from build123d import *

# Parameters (mm, degrees)
F0_W          = 70
F0_H          = 50
F1_DEPTH      = 130
F1_DEPTH_BACK = 70
F3_DEPTH      = 3


with BuildPart() as f1:
    # F0 (on Front) → F1 (new body, two sides)
    with BuildSketch(Plane.XZ) as f1_sk:
        Rectangle(F0_W, F0_H)
    extrude(amount=F1_DEPTH)
    extrude(f1_sk.sketch, amount=-F1_DEPTH_BACK)

    # F2 (on face) → F3 (join)
    with BuildSketch(Plane.XY.offset(25)):
        Polygon((-20, -117.372043), (0, -117.372043), (19.486902, -117.372043), (19.486902, -97.372043), (17.486902, -97.372043), (17.486902, -115.372043), (1, -115.372043), (1, -97.372043), (-1, -97.372043), (-1, -115.372043), (-18, -115.372043), (-18, -97.372043), (-20, -97.372043), align=None)
        with BuildLine():
            Line((8.707276, -43.856528), (19.913864, -43.856528))
            Line((19.913864, -43.856528), (19.913864, -41.856528))
            Line((19.913864, -41.856528), (4.924431, -41.856528))
            ThreePointArc((4.924431, -41.856528), (4.807975, -38.322004), (5.569528, -34.868535))
            Line((5.569528, -34.868535), (19.913864, -25.94221))
            Line((19.913864, -25.94221), (19.913864, -23.94221))
            Line((19.913864, -23.94221), (16.171332, -26.208643))
            ThreePointArc((16.171332, -26.208643), (16.198489, -26.228568), (16.225597, -26.24856))
            ThreePointArc((16.225597, -26.24856), (16.190659, -26.233277), (16.155661, -26.218133))
            Line((16.155661, -26.218133), (4.924431, -33.019635))
            ThreePointArc((4.924431, -33.019635), (-12.74275, -26.189347), (-19.573038, -43.856528))
            Line((-19.573038, -43.856528), (8.220368, -43.856528))
            ThreePointArc((8.220368, -43.856528), (8.255555, -43.764356), (8.290131, -43.671953))
            ThreePointArc((8.290131, -43.671953), (8.497604, -43.766725), (8.707276, -43.856528))
        make_face()
        with BuildLine():
            ThreePointArc((-17.680509, -41.856528), (-7.511621, -26.91543), (2.657267, -41.856528))
            Line((2.657267, -41.856528), (-17.680509, -41.856528))
        make_face(mode=Mode.SUBTRACT)
        with BuildLine():
            Line((-17.549662, 0), (-19.378563, 0))
            ThreePointArc((-19.378563, 0), (0.781648, -24.935632), (20.941859, 0))
            Line((20.941859, 0), (19.112958, 0))
            ThreePointArc((19.112958, 0), (0.781648, -23.151189), (-17.549662, 0))
        make_face()
        with BuildLine():
            Line((-19.573038, -68.369687), (0.426962, -68.369687))
            Line((0.426962, -68.369687), (19.913864, -68.369687))
            Line((19.913864, -68.369687), (19.913864, -48.369687))
            Line((19.913864, -48.369687), (17.913864, -48.369687))
            Line((17.913864, -48.369687), (17.913864, -66.369687))
            Line((17.913864, -66.369687), (1.426962, -66.369687))
            Line((1.426962, -66.369687), (1.426962, -48.838545))
            ThreePointArc((1.426962, -48.838545), (1.335768, -48.785469), (1.244992, -48.731682))
            ThreePointArc((1.244992, -48.731682), (0.956479, -48.554269), (0.672499, -48.369687))
            Line((0.672499, -48.369687), (-0.573038, -48.369687))
            Line((-0.573038, -48.369687), (-0.573038, -66.369687))
            Line((-0.573038, -66.369687), (-17.573038, -66.369687))
            Line((-17.573038, -66.369687), (-17.573038, -48.369687))
            Line((-17.573038, -48.369687), (-19.573038, -48.369687))
            Line((-19.573038, -48.369687), (-19.573038, -68.369687))
        make_face()
        Polygon((-20, -91.874998), (-20, -93.874998), (19.486902, -93.874998), (19.486902, -91.874998), (-15.315908, -91.874998), (19.486902, -73.169678), (19.486902, -71.169678), (-20, -71.169678), (-20, -73.169678), (14.462528, -73.169678), align=None)
        with BuildLine():
            add(Edge.make_bspline(
                [(19.94747, 13.162938), (19.94747, 34.677407), (-9.973735, 23.920172), (-39.89494, 13.162938), (-9.973735, 2.405704), (19.94747, -8.351531), (19.94747, 13.162938)],
                knots=[0, 0, 0, 2.094395, 2.094395, 4.18879, 4.18879, 6.283185, 6.283185, 6.283185], degree=2, weights=[1, 0.5, 1, 0.5, 1, 0.5, 1]))
        make_face()
        with BuildLine():
            add(Edge.make_bspline(
                [(17.490629, 13.162938), (17.490629, 30.363455), (-8.745315, 21.763196), (-34.981258, 13.162938), (-8.745315, 4.562679), (17.490629, -4.037579), (17.490629, 13.162938)],
                knots=[0, 0, 0, 2.094395, 2.094395, 4.18879, 4.18879, 6.283185, 6.283185, 6.283185], degree=2, weights=[1, 0.5, 1, 0.5, 1, 0.5, 1]))
        make_face(mode=Mode.SUBTRACT)
        Polygon((-18.922255, 27.677938), (20.941859, 27.678886), (21.023758, 29.677209), (-18.976242, 29.677209), align=None)
        Polygon((-19.378563, 34.858465), (-19.378563, 32.858465), (20.108339, 32.858465), (20.108339, 34.858465), (-14.694471, 34.858465), (20.108339, 53.563785), (20.108339, 55.563785), (-19.378563, 55.563785), (-19.378563, 53.563785), (15.083965, 53.563785), align=None)
    extrude(amount=F3_DEPTH)


solid = f1.part
Input: part model. Units: mm. Frame: model coordinates. A direction names the side the tool comes from. Give positions to 0.01 mm unless a question says otherwise; leave off trailing zeros. Loops run counter-clockwise (first coordinate to the right, second up) from the corner with the lowest first, then second, coordinate; pieces in that order, holes last. Notation, with made-up numbers: (31.5, -38.5) -> (84.5, -38.5) arc R28 ccw to (84.5, -11.5) -> close; hole circle Ø4 at (63, 47). An arc over 180 degrees is marked (long way). Answer as a JSON object with one key per item and string values. Group by question number.
Item 1: Pull-direction query (X, two-part tool) for faces 1 (the flat face through (0, 43, 28)), 2 (the flat face through (-8, -36, 25)), 3 (the flat face through (12.64, -30.47, 26.48)); classes: released by +X, released by -X, zero draft, split by the parting line, or undercut.
Item 2: Reachability of faces 4 (the flat face through (1.842, -82.653, 26.479)), 5 (the flat face through (35, -31, 0)), 6 (the flat face through (-2.527, -82.391, 26.479)), 7 (the cylindrical face through (1.257, -23.145, 26.479)), 8 (the flat face through (0, -130, 0)) from +Z, -Z, +X, -X, +Y, -Y: full face, straight path, thin tool, end or side. Return the list, or none.
Item 3: Pin query (flat end, axial travel): P1, Ø2.5, axis at y = -112.5, z = 26.5, coming from the +X side; P2, Ø1, axis at y = 34.5, z = 26.5, coming from the -X side; P3, Ø0.9, axis at x = 2, z = 26.5, coming from the +Y side; P4, Ø2.5, axis at y = -103, z = 26, coming from the +X side. Return the tip coordinate at first contact, or that it passes through.
Item 4: Cut plane A-A, the plane y = -105. Return the cut outline in (x, z).
Item 5: Line query: probe 1 along Z at (x, y) = (-22, -14.5). Output: solid intervals per line, ascending.
Checks:
{
 "1": {"face 1": "zero draft", "face 2": "undercut", "face 3": "released by +X"},
 "2": {"face 4": "+Z, +X", "face 5": "+Z, -Z, +X, +Y, -Y", "face 6": "+Z, -X", "face 7": "+Z", "face 8": "+Z, -Z, +X, -X, -Y"},
 "3": {"P1": "stops at x = 19.49", "P2": "stops at x = -19.38", "P3": "stops at y = 55.56", "P4": "stops at x = 35"},
 "4": {"outline": "(-35, -25) -> (35, -25) -> (35, 25) -> (19.49, 25) -> (19.49, 28) -> (17.49, 28) -> (17.49, 25) -> (1, 25) -> (1, 28) -> (-1, 28) -> (-1, 25) -> (-18, 25) -> (-18, 28) -> (-20, 28) -> (-20, 25) -> (-35, 25) -> close"},
 "5": {"probe 1": "z = -25 to 25"}
}
